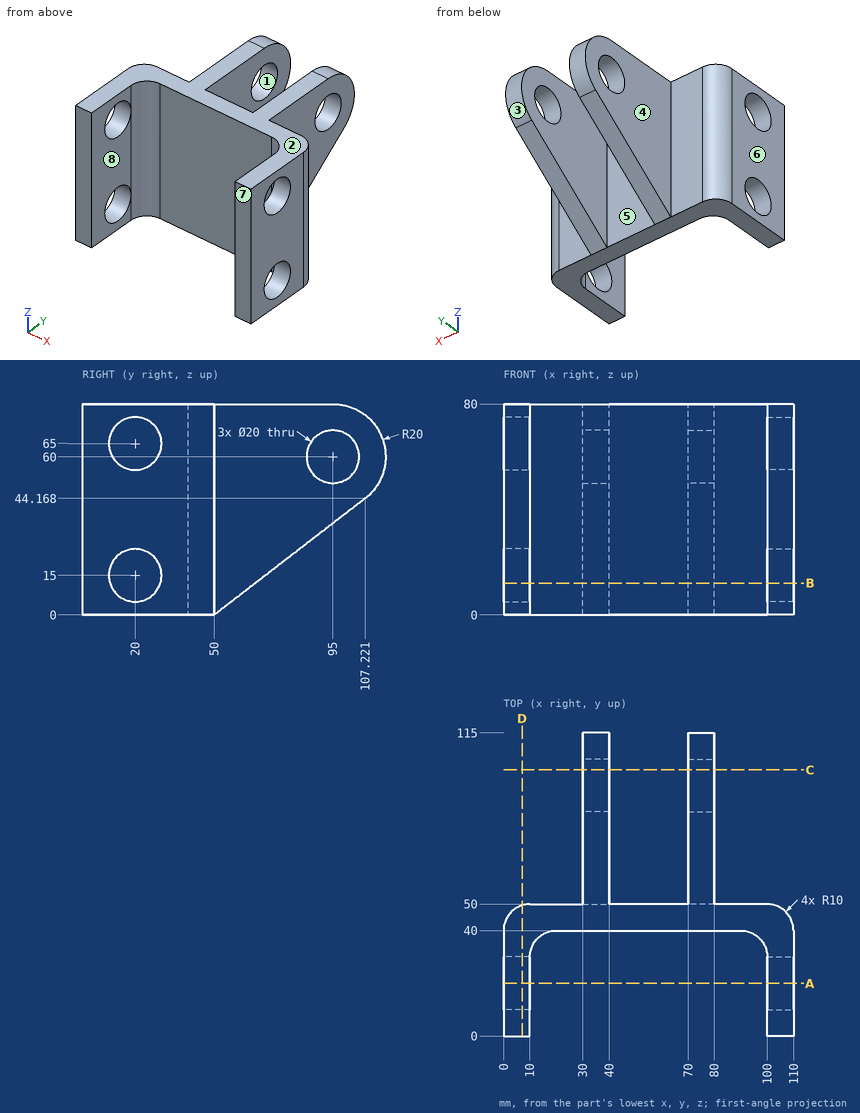
Input: dimensioned drawing with shaded views. Units: mm. Origin: part minimum x, y, z. A direction names the side the tool comes from. Coordinates: 2 decimals unless noted, no trailing zeros. Order: outer loops, then holes, each group sorted by start corner. A loop starts at its lowest first (then second) coordinate and runs counter-clockwise, first axis right, second up.
(1) Draft query along Y for the marked faces 1, 2 and 3. Return one class per face: pulls with the +Y half, pulls with the -Y half, needs draft (parallel to the pull), parting line crosses it, or undercut.
(2) Section query D-D (x = 7). Return the cut outline in (y, z).
(3) Section query B-B (z = 12). Return the cut outline in (x, y), plus the area to 3 significant figures.
(4) Material intervals for probe 1 along X at (y, z) = (72.5, 33.5); probe 2 along X at (y, z) = (26.5, 33.5); probe 3 along Y at (x, z) = (52, 43.5), sorted ascending.
(5) First-contact query: pin 1 (16 mm diameter, centred on y = 20, z = 15, fed in from -X); pin 2 (15 mm diameter, centred on x = 58, z = 32, fed in from +Y); pin 3 (1.5 mm diameter, centred on y = 58, z = 56.5, fed in from -X); pin 4 (23 mm diameter, centred on y = 20, z = 65, fed in from -X). Flat tips, straight axial feed; report the tip coordinate or a pass-through.
(6) Section query A-A (y = 20). Return the cut outline in (x, z), plus the area to 3 significant figures.
(7) Section query C-C (y = 101). Return the cut outline in (x, z), plus the area to 3 significant figures.
(8) Access query for the marked faces 4, 5, 6, 7 and 8. Directions: +Z, -Z, +X, -X, +Y, -Y. A direction counts if a zero-diameter tool reaches every point of the face in a straight line with its end or side. Return the directions, or none.
Solution:
1. face 1: undercut
1. face 2: needs draft
1. face 3: pulls with the +Y half
2. outline: (0, 0) - (49.54, 0) - (49.54, 80) - (0, 80) - close; hole circle Ø20 at (20, 15); hole circle Ø20 at (20, 65)
3. outline: (0, 0) - (10, 0) - (10, 10.46) - (0, 10.46) - close; (0, 29.54) - (10, 29.54) - (10, 30) arc R10 cw to (20, 40) - (90, 40) arc R10 cw to (100, 30) - (100, 29.54) - (110, 29.54) - (110, 40) arc R10 ccw to (100, 50) - (80, 50) - (80, 65.55) - (70, 65.55) - (70, 50) - (40, 50) - (40, 65.55) - (30, 65.55) - (30, 50) - (10, 50) arc R10 ccw to (0, 40) - close; (100, 0) - (110, 0) - (110, 10.46) - (100, 10.46) - close
3. area: 1,830 mm2
4. probe 1: x = 30 to 40, 70 to 80
4. probe 2: x = 0 to 10, 100 to 110
4. probe 3: y = 40 to 50
5. pin 1: passes through
5. pin 2: stops at y = 50
5. pin 3: stops at x = 30
5. pin 4: stops at x = 0
6. outline: (0, 0) - (10, 0) - (10, 5) - (0, 5) - close; (0, 25) - (10, 25) - (10, 55) - (0, 55) - close; (0, 75) - (10, 75) - (10, 80) - (0, 80) - close; (100, 0) - (110, 0) - (110, 5) - (100, 5) - close; (100, 25) - (110, 25) - (110, 55) - (100, 55) - close; (100, 75) - (110, 75) - (110, 80) - (100, 80) - close
6. area: 800 mm2
7. outline: (30, 39.37) - (40, 39.37) - (40, 52) - (30, 52) - close; (30, 68) - (40, 68) - (40, 79.08) - (30, 79.08) - close; (70, 39.37) - (80, 39.37) - (80, 52) - (70, 52) - close; (70, 68) - (80, 68) - (80, 79.08) - (70, 79.08) - close
7. area: 474 mm2
8. face 4: +Z, -Z, -X, +Y
8. face 5: +Z, -Z, +Y
8. face 6: +Z, -Z, -X, +Y, -Y
8. face 7: +Z, -Z, +X, -X, -Y
8. face 8: +Z, -Z, -Y
